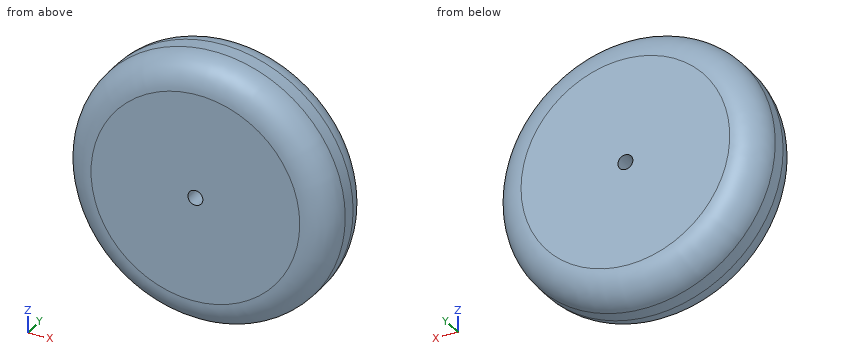
from build123d import *

# Parameters (mm, degrees)
SKETCH1_R                = 114.3
BOSS_EXTRUDE1_DEPTH      = 31.75
BOSS_EXTRUDE1_DEPTH_BACK = 31.75
FILLET1_R                = 25.4
SKETCH2_R                = 6.35
CUT_EXTRUDE1_DEPTH       = 107.188


with BuildPart() as part:
    # Sketch1 → Boss-Extrude1 (new body, two sides)
    with BuildSketch(Plane(origin=(0, 0, 0), x_dir=(1, 0, 0), z_dir=(0, 1, 0))) as boss_extrude1_sk:
        Circle(SKETCH1_R)
    extrude(amount=BOSS_EXTRUDE1_DEPTH)
    extrude(boss_extrude1_sk.sketch, amount=-BOSS_EXTRUDE1_DEPTH_BACK)

    # Fillet1
    fillet1_edges = [part.edges().sort_by_distance(p)[0] for p in [
        (-114.3, -31.75, 0),
        (-114.3, 31.75, 0),
    ]]
    fillet(fillet1_edges, radius=FILLET1_R)

    # Sketch2 → Cut-Extrude1 (cut)
    with BuildSketch(Plane(origin=(0, 31.75, 0), x_dir=(1, 0, 0), z_dir=(0, 1, 0))):
        Circle(SKETCH2_R)
    extrude(amount=-CUT_EXTRUDE1_DEPTH, mode=Mode.SUBTRACT)


solid = part.part
Can you work these out from the model? Positions are in its coordinate system, mm. Give positions to 0.01 mm unless a question says otherwise; leave off trailing zeros. Order: outer loops, then holes, each group sorted by start corner. A loop starts at its lowest first (then second) coordinate and runs counter-clockwise, first axis right, second up. Notation, with made-up numbers: M 46,-11 L 75,-11 A10 ccw 75,-6 Z; hole C 58.5,-7.5 d8. An arc over 180 degrees is marked long. Use one line per item in the form item = value. Start each with the question number.
Item 1: If we section it at C-C (y = -19.5): Write out the boundary of the cut face in (x, z), then the cut area to 3 significant figures.
Item 2: If we section it at B-B (z = 0): Write out the boundary of the cut face in (x, y), then the cut area to 3 significant figures.
Item 3: If we section it at A-A (x = 0): Write out the boundary of the cut face in (y, z).
Item 4: Will these pins go through, and if not, where does the flat tip stop? pin 1 Ø16.5 at (x, z) = (0, 0) entering from +Y; pin 2 Ø1 at (x, y) = (4, 17.5) entering from -Z; pin 3 Ø4 at (y, z) = (10.5, -41.5) entering from -X; pin 4 Ø10 at (x, y) = (54, 11) entering from +Z.
Item 5: If I drill on line 1 along Z through (x, y) = (0, 0); line 2 along Z through (x, y) = (0, 18), over which ranges is the centre line in solid material (lowest first)?
Outcome:
q1.outline = C 0,0 d221.26; hole C 0,0 d12.7
q1.area = 38,300 mm2
q2.outline = M -114.3,-6.35 A25.4 ccw -88.9,-31.75 L -6.35,-31.75 L -6.35,31.75 L -88.9,31.75 A25.4 ccw -114.3,6.35 Z; M 6.35,-31.75 L 88.9,-31.75 A25.4 ccw 114.3,-6.35 L 114.3,6.35 A25.4 ccw 88.9,31.75 L 6.35,31.75 Z
q2.area = 13,200 mm2
q3.outline = M -31.75,-88.9 A25.4 ccw -6.35,-114.3 L 6.35,-114.3 A25.4 ccw 31.75,-88.9 L 31.75,-6.35 L -31.75,-6.35 Z; M -31.75,6.35 L 31.75,6.35 L 31.75,88.9 A25.4 ccw 6.35,114.3 L -6.35,114.3 A25.4 ccw -31.75,88.9 Z
q4.pin_1 = 31.75
q4.pin_2 = -111.89
q4.pin_3 = -106.96
q4.pin_4 = 102.94
q5.line_1 = -114.3 to -6.35, 6.35 to 114.3
q5.line_2 = -111.47 to -6.35, 6.35 to 111.47
